Work out the finished part from the listing and answer in its coordinate system (mm). A direction names the side the tool comes from. Give positions to 0.01 mm unless a question says otherwise; leave off trailing zeros. Loops run counter-clockwise (first coordinate to the right, second up) from the corner with the lowest first, then second, coordinate; pieces in that order, holes last. Notation, with made-up numbers: (44, 3) - (83, 3) arc R18 cw to (83, 24) - close; hole circle Ø2 at (-34, 50.5). An arc over 180 degrees is marked (long way). One line per question, with ' | ' between items.
from build123d import *

# Parameters (mm, degrees)
SKETCH1_R                     = 2.75
BOSS_EXTRUDE1_DEPTH           = 10
SKETCH3_R                     = 2
CUT_EXTRUDE1_DEPTH            = 32.5
ESBO_O1_R                     = 2
RESSALTO_EXTRUS_O2_DEPTH      = 13
RESSALTO_EXTRUS_O2_DEPTH_BACK = 3
CORTE_EXTRUS_O1_DEPTH         = 5
FILETE1_R                     = 0.2
FILETE2_R                     = 0.25
CHAMFER_1_SIZE                = 0.3
FILLET_1_R                    = 0.3


with BuildPart() as part:
    # Sketch1 → Boss-Extrude1 (new body)
    with BuildSketch(Plane(origin=(0, 0, 0), x_dir=(1, 0, 0), z_dir=(0, 1, 0))):
        with BuildLine():
            Line((21.5, 0.100660355), (21.5, -0.100660355))
            ThreePointArc((21.5, -0.100660355), (20.891804651, -2.072326113), (19.278590937, -3.35875876))
            Line((19.278590937, -3.35875876), (10, -7))
            Line((10, -7), (10, -14))
            Line((10, -14), (0.5, -14))
            Line((0.5, -14), (0.5, -4.974937186))
            ThreePointArc((0.5, -4.974937186), (0, 5), (-0.5, -4.974937186))
            Line((-0.5, -4.974937186), (-0.5, -14))
            Line((-0.5, -14), (-10, -14))
            Line((-10, -14), (-10, -7))
            Line((-10, -7), (-19.278590937, -3.35875876))
            ThreePointArc((-19.278590937, -3.35875876), (-20.891804651, -2.072326113), (-21.5, -0.100660355))
            Line((-21.5, -0.100660355), (-21.5, 0.100660355))
            ThreePointArc((-21.5, 0.100660355), (-20.881804225, 2.086914218), (-19.245597481, 3.371514512))
            Line((-19.245597481, 3.371514512), (-3.558849946, 9.345297591))
            ThreePointArc((-3.558849946, 9.345297591), (0, 10), (3.558849946, 9.345297591))
            Line((3.558849946, 9.345297591), (19.245597481, 3.371514512))
            ThreePointArc((19.245597481, 3.371514512), (20.881804225, 2.086914218), (21.5, 0.100660355))
        make_face()
        with Locations(Location((-16, 0, 0), (0, 0, 270))):  # turned: the seam where the file's is
            Circle(SKETCH1_R, mode=Mode.SUBTRACT)
        with Locations(Location((16, 0, 0), (0, 0, 270))):  # turned: the seam where the file's is
            Circle(SKETCH1_R, mode=Mode.SUBTRACT)
    extrude(amount=BOSS_EXTRUDE1_DEPTH)

    # Sketch3 → Cut-Extrude1 (cut, through all)
    with BuildSketch(Plane(origin=(10, 0, 0), x_dir=(0, 0, -1), z_dir=(1, 0, 0))):
        with Locations((-10.5, 5)):
            Circle(SKETCH3_R)
    extrude(amount=-CUT_EXTRUDE1_DEPTH, mode=Mode.SUBTRACT)

    # Esboço1 → Ressalto-extrusão2 (add, two sides)
    with BuildSketch(Plane.ZY.offset(-10)) as ressalto_extrus_o2_sk:
        with Locations(Location((10.5, 5, 0), (0, 0, 180))):  # turned: the seam where the file's is
            Circle(ESBO_O1_R)
    extrude(amount=RESSALTO_EXTRUS_O2_DEPTH)
    extrude(ressalto_extrus_o2_sk.sketch, amount=-RESSALTO_EXTRUS_O2_DEPTH_BACK)

    # Esboço2 → Corte-extrusão1 (cut)
    with BuildSketch(Plane.ZY.offset(-13)):
        Polygon((10.90776936, 4.293722751), (11.315538719, 5), (10.90776936, 5.706277249), (10.09223064, 5.706277249), (9.684461281, 5), (10.09223064, 4.293722751), align=None)
    extrude(amount=CORTE_EXTRUS_O1_DEPTH, mode=Mode.SUBTRACT)

    # Filete1
    filete1_edges = [part.edges().sort_by_distance(p)[0] for p in [
        (13, 5, 12.5),
        (13, 4.646861376, 11.11165404),
        (13, 4.293722751, 10.5),
        (13, 4.646861376, 9.88834596),
        (13, 5.353138624, 9.88834596),
        (13, 5.706277249, 10.5),
        (13, 5.353138624, 11.11165404),
    ]]
    fillet(filete1_edges, radius=FILETE1_R)

    # Filete2
    filete2_edges = [part.edges().sort_by_distance(p)[0] for p in [
        (-3, 5, 12.5),
    ]]
    fillet(filete2_edges, radius=FILETE2_R)

    # Фаска1
    chamfer_1_edges = [part.edges().sort_by_distance(p)[0] for p in [
        (0, 0, -5),
        (-16, 0, -2.75),
        (0, 10, -5),
        (-16, 10, -2.75),
        (16, 0, -2.75),
        (16, 10, -2.75),
    ]]
    chamfer(chamfer_1_edges, length=CHAMFER_1_SIZE)

    # Скругление1
    fillet_1_edges = [part.edges().sort_by_distance(p)[0] for p in [
        (10, 5, 14),
        (-10, 5, 14),
    ]]
    fillet(fillet_1_edges, radius=FILLET_1_R)


solid = part.part
1. Consider L1, parallel to X at y = 2.5, z = 0; L2, parallel to X at y = 2.5, z = 9; L3, parallel to X at y = 8.5, z = -1.75. Determine where each line is inside the solid, lowest interval first.
Evaluation:
L1: -21.5 to -18.75, -13.25 to -5, 5 to 13.25, 18.75 to 21.5 | L2: -10 to -0.5, 0.5 to 10 | L3: -21.09 to -18.12, -13.88 to -4.68, 4.68 to 13.88, 18.12 to 21.09
2. Find section A-A on z = 7.75. Write down the section's boundary in (x, y).
Evaluation:
outline: (-10, 0) - (-0.5, 0) - (-0.5, 10) - (-10, 10) - close; (0.5, 0) - (10, 0) - (10, 10) - (0.5, 10) - close
3. Flat-ended cylindrical pins translate along their axes: pin 1 (5 mm diameter, centred on y = 5, z = 10.5, fed in from +X); pin 2 (7 mm diameter, centred on x = 16, z = 0, fed in from +Y); pin 3 (1.5 mm diameter, centred on x = 12, y = 1.5, fed in from -Z); pin 4 (0.9 mm diameter, centred on x = 11.5, z = 10.5, fed in from +Y). Find the tip coordinate at first contact, or state that the pin passes through.
Evaluation:
pin 1: x = 13 | pin 2: y = 10 | pin 3: z = -6.42 | pin 4: y = 7
4. Determine the mould class of faces 4 (the flat face through (10.4, 5.706, 10.5)), 5 (the flat face through (5, 0, 4)), 6 (the cylindrical face through (0, 5, -10)) for opening direction Z: +Z half, -Z half, draft (parallel to the pull), parting line (faces both ways), or undercut.
Evaluation:
face 4: undercut | face 5: draft | face 6: -Z half
5. Which of the six approach directions +Z, -Z, +X, -X, +Y, -Y give full straight-line access (tool end or side, diameter ignored) to faces 1 (the flat face through (13, 5.8, 9.7)), 2 (the flat face through (0.5, 3.8, 8.5)), 3 (the flat face through (8, 5, 10))?
Evaluation:
face 1: +Z, +X, +Y, -Y | face 2: none | face 3: +X
6. Find section B-B on y = 8.5. Write down the section's boundary in (x, z).
Evaluation:
outline: (-21.5, -0.1) arc R3.5 ccw to (-19.25, -3.37) - (-3.56, -9.35) arc R10 ccw to (3.56, -9.35) - (19.25, -3.37) arc R3.5 ccw to (21.5, -0.1) - (21.5, 0.1) arc R3.5 ccw to (19.28, 3.36) - (10, 7) - (10, 13.7) arc R0.3 ccw to (9.7, 14) - (0.5, 14) - (0.5, 4.97) arc R5 cw (long way) to (-0.5, 4.97) - (-0.5, 14) - (-9.7, 14) arc R0.3 ccw to (-10, 13.7) - (-10, 7) - (-19.28, 3.36) arc R3.5 ccw to (-21.5, 0.1) - close; hole circle Ø5.5 at (-16, 0); hole circle Ø5.5 at (16, 0)
7. Find section C-C on x = 0. Write down the section's boundary in (y, z).
Evaluation:
outline: (0, -10) - (10, -10) - (10, -5.3) - (9.7, -5) - (0.3, -5) - (0, -5.3) - close; circle Ø4 at (5, 10.5)
